Input: dimensioned drawing with shaded views. Units: mm. Origin: part minimum x, y, z. A direction names the side the tool comes from. Coordinates: 2 decimals unless noted, no trailing zeros. Order: outer loops, then holes, each group sorted by start corner. A loop starts at its lowest first (then second) coordinate and runs counter-clockwise, first axis right, second up. Notation, with made-up numbers: (-35, 78.25) - (-7, 78.25) arc R32 ccw to (-7, 117.25) - close; hole circle Ø8 at (59, 47.25). An arc over 180 degrees is marked (long way). Answer as CSV lines item,"result". Start each with the question number.
Item 1: Section A-A (y = 25.4). State how many separate pieces and enclosed holes the cut face has, and give its area (3 significant figures).
Item 2: Section D-D (z = 48.5). Output: boundary loops of the cut face in (x, y), and give its area (3 significant figures).
Item 3: Material intervals for line 1 along X through (y, z) = (25, 4); line 2 along X through (y, z) = (34, 42) (1 decimal); line 3 along Y through (x, z) = (114, 5), sorted ascending.
Item 4: Access query for the marked faces 5, 6 and 7. Directions: +Z, -Z, +X, -X, +Y, -Y. A direction counts if a zero-diameter tool reaches every point of the face in a straight line with its end or side. Return the directions, or none.
Item 5: Draft query along Y for the marked faces 1, 2, 3 and 4. Return one class per face: +Y half, -Y half, draft (parallel to the pull), parting line (faces both ways), or undercut.
Item 6: Section B-B (x = 114.3). Output: boundary loops of the cut face in (y, z).
Item 7: First-contact query: pin 1 (23 mm diameter, centred on x = 66.548, z = 41.148, fed in from +Y); pin 2 (23 mm diameter, centred on y = 27, z = 26, fed in from -X); pin 3 (5 mm diameter, centred on y = 29.5, z = 28, fed in from +X); pin 4 (3 mm diameter, centred on x = 108, y = 36, fed in from +Z). Flat tips, straight axial feed; report the tip coordinate or a pass-through.
Item 8: Section C-C (z = 9.5). Output: boundary loops of the cut face in (x, y).
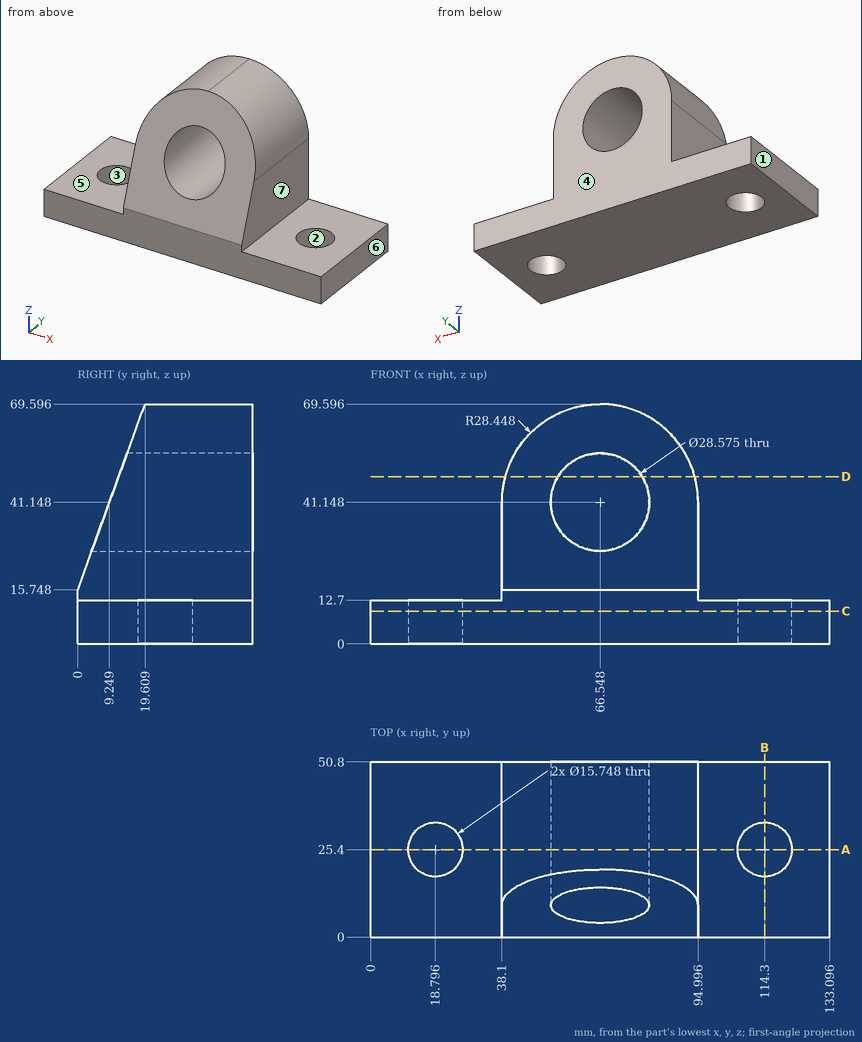
Determined:
1,separate pieces,"3"
1,enclosed holes,"1"
1,area,"3,540 mm^2"
2,outline,"(39.07, 11.93) - (54.3, 11.93) - (54.3, 50.8) - (39.07, 50.8) - close; (78.8, 11.93) - (94.03, 11.93) - (94.03, 50.8) - (78.8, 50.8) - close"
2,area,"1,180 mm^2"
3,line 1,"x = 0 to 10.93, 26.66 to 106.44, 122.16 to 133.1"
3,line 2,"x = 38.1 to 52.3, 80.8 to 95"
3,line 3,"y = 0 to 17.53, 33.27 to 50.8"
4,face 5,"+Z, -X, +Y, -Y"
4,face 6,"+Z, -Z, +X, +Y, -Y"
4,face 7,"+Z, +X, +Y, -Y"
5,face 1,"draft"
5,face 2,"undercut"
5,face 3,"undercut"
5,face 4,"+Y half"
6,outline,"(0, 0) - (17.53, 0) - (17.53, 12.7) - (0, 12.7) - close; (33.27, 0) - (50.8, 0) - (50.8, 12.7) - (33.27, 12.7) - close"
7,pin 1,"passes through"
7,pin 2,"stops at x = 38.1"
7,pin 3,"stops at x = 95"
7,pin 4,"stops at z = 12.7"
8,outline,"(0, 0) - (133.1, 0) - (133.1, 50.8) - (0, 50.8) - close; hole circle Ø15.75 at (18.8, 25.4); hole circle Ø15.75 at (114.3, 25.4)"
